from build123d import *

# Parameters (mm, degrees)
ESBO_O1_R                = 4.05
ESBO_O1_R_2              = 7.75
RESSALTO_EXTRUS_O1_DEPTH = 6
RESSALTO_EXTRUS_O2_START = -1
ESBO_O2_R                = 7.75
ESBO_O2_R_2              = 7
RESSALTO_EXTRUS_O2_DEPTH = 1


with BuildPart() as part:
    # Esboço1 → Ressalto-extrusão1 (new body)
    with BuildSketch(Plane(origin=(0, 0, 0), x_dir=(1, 0, 0), z_dir=(0, 1, 0))):
        with BuildLine():
            Line((-33.07179677, 4), (-16.645194502, 4))
            ThreePointArc((-16.645194502, 4), (-12.424283231, 4.934465926), (-8.992231512, 7.563218391))
            ThreePointArc((-8.992231512, 7.563218391), (0, 11.75), (8.992231512, 7.563218391))
            ThreePointArc((8.992231512, 7.563218391), (12.424283231, 4.934465926), (16.645194502, 4))
            Line((16.645194502, 4), (33.07179677, 4))
            ThreePointArc((33.07179677, 4), (48, 0), (33.07179677, -4))
            Line((33.07179677, -4), (16.645194502, -4))
            ThreePointArc((16.645194502, -4), (12.424283231, -4.934465926), (8.992231512, -7.563218391))
            ThreePointArc((8.992231512, -7.563218391), (0, -11.75), (-8.992231512, -7.563218391))
            ThreePointArc((-8.992231512, -7.563218391), (-12.424283231, -4.934465926), (-16.645194502, -4))
            Line((-16.645194502, -4), (-33.07179677, -4))
            ThreePointArc((-33.07179677, -4), (-48, 0), (-33.07179677, 4))
        make_face()
        with Locations(Location((40, 0, 0), (0, 0, 270))):
            Circle(ESBO_O1_R, mode=Mode.SUBTRACT)
        with Locations(Location((-40, 0, 0), (0, 0, 270))):
            Circle(ESBO_O1_R, mode=Mode.SUBTRACT)
        with Locations(Location((0, 0, 0), (0, 0, 270))):
            Circle(ESBO_O1_R_2, mode=Mode.SUBTRACT)
    extrude(amount=RESSALTO_EXTRUS_O1_DEPTH)

    # Esboço2 → Ressalto-extrusão2 (add)
    with BuildSketch(Plane(origin=(0, 6, 0), x_dir=(1, 0, 0), z_dir=(0, 1, 0)).offset(RESSALTO_EXTRUS_O2_START)):
        with Locations(Location((0, 0, 0), (0, 0, 270))):
            Circle(ESBO_O2_R)
        with Locations(Location((0, 0, 0), (0, 0, 270))):
            Circle(ESBO_O2_R_2, mode=Mode.SUBTRACT)
    extrude(amount=RESSALTO_EXTRUS_O2_DEPTH)


solid = part.part
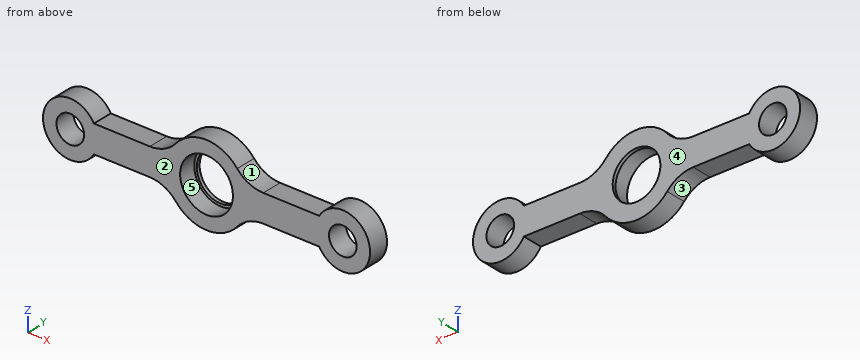
CAD build for the part. Positions are in the model's coordinates, mm. Face numbers are marked on the shaded views. A direction names the side the tool comes from. Coordinates: 2 decimals unless noted, no trailing zeros. Loops run counter-clockwise (first coordinate to the right, second up) from the corner with the lowest first, then second, coordinate; pieces in that order, holes last. Notation, with made-up numbers: (61, -8.75) - (77, -8.75) arc R3 ccw to (77, -4.75) - close; hole circle Ø3 at (3.5, 28). An arc over 180 degrees is marked (long way). Write item = value, one per line. Start each with the question number.
Q1. Pull direction X, two halves, no side cores. Call the marked faces 4 and 5: pulls with the +X half, pulls with the -X half, needs draft (parallel to the pull), parting line crosses it, or undercut.
Q2. Cut at C-C, the plane x = -40. List the corners of the cut face in (y, z).
Q3. Cut at A-A, the plane z = 0. List the corners of the cut face in (x, y).
Q4. Cut at B-B, the plane y = 4.1. List the corners of the cut face in (x, z), then the cut area to 3 significant figures.
Q5. Cut at D-D, the plane x = 0. List the corners of the cut face in (y, z).
Q6. Which spindle directions (+Z, -Z, +X, -X, +Y, -Y) get a long thin tool onto all of the face, cutting with end or side? Do the marked faces 1, 2 and 3. Say none if no direction does.
Q7. Drill centre lines: L1, parallel to X at y = 2.7, z = 0; L2, parallel to X at y = 0.85, z = 5.75; L3, parallel to Z at x = -23.5, y = 4.8. Where is each one in solid material? Low to high.
Q8. Flat gauge pins, fed straight in: pin 1 Ø3 at (x, y) = (-21, 3) entering from -Z; pin 2 Ø1.8 at (x, y) = (28.5, 4) entering from +Z; pin 3 Ø1 at (y, z) = (3.5, 2) entering from +X. Where does each tip first touch, or does it go through?
Computed:
q1.face_4 = needs draft
q1.face_5 = undercut
q2.outline = (0, -8) - (6, -8) - (6, -4.05) - (0, -4.05) - close; (0, 4.05) - (6, 4.05) - (6, 8) - (0, 8) - close
q3.outline = (-48, 0) - (-44.05, 0) - (-44.05, 6) - (-48, 6) - close; (-35.95, 0) - (-7.75, 0) - (-7.75, 5) - (-7, 5) - (-7, 6) - (-35.95, 6) - close; (7, 5) - (7.75, 5) - (7.75, 0) - (35.95, 0) - (35.95, 6) - (7, 6) - close; (44.05, 0) - (48, 0) - (48, 6) - (44.05, 6) - close
q4.outline = (-33.07, -4) - (-16.65, -4) arc R10 cw to (-8.99, -7.56) arc R11.75 ccw to (8.99, -7.56) arc R10 cw to (16.65, -4) - (33.07, -4) arc R8 ccw (long way) to (33.07, 4) - (16.65, 4) arc R10 cw to (8.99, 7.56) arc R11.75 ccw to (-8.99, 7.56) arc R10 cw to (-16.65, 4) - (-33.07, 4) arc R8 ccw (long way) to start; hole circle Ø8.1 at (-40, 0); hole circle Ø15.5 at (0, 0); hole circle Ø8.1 at (40, 0)
q4.area = 894 mm²
q5.outline = (0, -11.75) - (6, -11.75) - (6, -7) - (5, -7) - (5, -7.75) - (0, -7.75) - close; (0, 7.75) - (5, 7.75) - (5, 7) - (6, 7) - (6, 11.75) - (0, 11.75) - close
q6.face_1 = +Z, +Y, -Y
q6.face_2 = +Z, -Z, +X, -X, -Y
q6.face_3 = -Z, +Y, -Y
q7.L1 = -48 to -44.05, -35.95 to -7.75, 7.75 to 35.95, 44.05 to 48
q7.L2 = -45.56 to -34.44, -10.99 to -5.2, 5.2 to 10.99, 34.44 to 45.56
q7.L3 = -4 to 4
q8.pin_1 = -4
q8.pin_2 = 4
q8.pin_3 = 47.86
